The listing builds one solid part. Answer for the finished solid, in the listing's coordinates (mm). A direction names the side the tool comes from. Give positions to 0.01 mm unless a question says otherwise; leave off trailing zeros. Write each loop counter-clockwise with the first axis right and the second up, starting at its lowest first coordinate (ties: lowest second). Pieces come first, ordered by that corner, then holes. Notation, with made-up numbers: (43, 60) - (64, 60) arc R26 cw to (64, 99) - close; hole circle Ø4 at (14.25, 68.25). An arc over 180 degrees is marked (long way). Return JSON: item names as keys, results as strings.
from build123d import *

# Parameters (mm, degrees)
SKETCH1_W           = 340
SKETCH1_H           = 42.5
BOSS_EXTRUDE1_DEPTH = 41.5
SKETCH2_R           = 9.5
CUT_EXTRUDE1_DEPTH  = 10
SKETCH4_R           = 3.05
CUT_EXTRUDE3_DEPTH  = 301.787476707
CUT_EXTRUDE4_DEPTH  = 344.473796902


with BuildPart() as part:
    # Sketch1 → Boss-Extrude1 (new body)
    with BuildSketch(Plane(origin=(0, 0, 0), x_dir=(1, 0, 0), z_dir=(0, 1, 0))):
        with Locations((126.814516129, -4.284274194)):
            Rectangle(SKETCH1_W, SKETCH1_H)
    extrude(amount=BOSS_EXTRUDE1_DEPTH)

    # Sketch2 → Cut-Extrude1 (cut)
    with BuildSketch(Plane(origin=(0, 41.5, 0), x_dir=(1, 0, 0), z_dir=(0, 1, 0))):
        with Locations(Location((-5.685483871, -4.284274194, 0), (0, 0, 270))):
            Circle(SKETCH2_R)
        with Locations(Location((26.914516129, -4.284274194, 0), (0, 0, 270))):
            Circle(SKETCH2_R)
        with Locations(Location((59.514516129, -4.284274194, 0), (0, 0, 270))):
            Circle(SKETCH2_R)
        with Locations(Location((92.114516129, -4.284274194, 0), (0, 0, 270))):
            Circle(SKETCH2_R)
        with Locations(Location((124.714516129, -4.284274194, 0), (0, 0, 270))):
            Circle(SKETCH2_R)
        with Locations(Location((157.314516129, -4.284274194, 0), (0, 0, 270))):
            Circle(SKETCH2_R)
        with Locations(Location((189.914516129, -4.284274194, 0), (0, 0, 270))):
            Circle(SKETCH2_R)
        with Locations(Location((222.514516129, -4.284274194, 0), (0, 0, 270))):
            Circle(SKETCH2_R)
        with Locations(Location((255.114516129, -4.284274194, 0), (0, 0, 270))):
            Circle(SKETCH2_R)
    extrude(amount=-CUT_EXTRUDE1_DEPTH, mode=Mode.SUBTRACT)

    # Sketch4 → Cut-Extrude3 (cut, through all)
    with BuildSketch(Plane(origin=(0, 41.5, 0), x_dir=(1, 0, 0), z_dir=(0, 1, 0))):
        with Locations(Location((286.814516129, 8.965725806, 0), (0, 0, 90))):
            Circle(SKETCH4_R)
        with Locations(Location((-33.185483871, -17.534274194, 0), (0, 0, 90))):
            Circle(SKETCH4_R)
    extrude(amount=-CUT_EXTRUDE3_DEPTH, mode=Mode.SUBTRACT)

    # Sketch3 → Cut-Extrude4 (cut, through all)
    with BuildSketch(Plane.ZY.offset(43.185483871)):
        with BuildLine():
            Line((-6.965725806, 41.5), (-16.965725806, 41.5))
            Line((-16.965725806, 41.5), (-16.965725806, 31.5))
            ThreePointArc((-16.965725806, 31.5), (-14.036793618, 38.571067812), (-6.965725806, 41.5))
        make_face()
        with BuildLine():
            ThreePointArc((-6.965725806, 0), (-14.036793618, 2.928932188), (-16.965725806, 10))
            Line((-16.965725806, 10), (-16.965725806, 0))
            Line((-16.965725806, 0), (-6.965725806, 0))
        make_face()
        with BuildLine():
            Line((25.534274194, 0), (25.534274194, 10))
            ThreePointArc((25.534274194, 10), (22.605342005, 2.928932188), (15.534274194, 0))
            Line((15.534274194, 0), (25.534274194, 0))
        make_face()
        with BuildLine():
            Line((25.534274194, 41.5), (15.534274194, 41.5))
            ThreePointArc((15.534274194, 41.5), (22.605342005, 38.571067812), (25.534274194, 31.5))
            Line((25.534274194, 31.5), (25.534274194, 41.5))
        make_face()
    extrude(amount=-CUT_EXTRUDE4_DEPTH, mode=Mode.SUBTRACT)


solid = part.part
Item 1: A cutting plane is placed at C-C on y = 36. Give the number of separate pieces and of enclosed holes in the cut face, then the cut area to 3 significant figures.
Answer below:
{"separate pieces": "1", "enclosed holes": "11", "area": "11,100 mm²"}
Item 2: For faces 5 (the face through (50.24, 36.57, 2.22)), 6 (the face through (-30.48, 21.04, 16.13)), determine the directions among +Z, -Z, +X, -X, +Y, -Y from which every point of the face is accessible in a straight line to the end or side of a thin tool.
Answer below:
{"face 5": "+Y", "face 6": "+Y, -Y"}
Item 3: Flat-ended cylindrical pins translate along their axes: P1, Ø5.5, axis at x = 220.5, z = 6.5, coming from the +Y side; P2, Ø1, axis at x = 256.5, y = 7.5, coming from the +Z side. Find the tip coordinate at first contact, or state that the pin passes through.
Answer below:
{"P1": "stops at y = 31.5", "P2": "stops at z = 25.33"}
Item 4: The mould has two halves that part along X. Classify faces 1 (the face through (124, 21, -16.966)), 2 (the face through (100.125, 36.57, 9.391)), 3 (the face through (-43.185, 20, 5)), 4 (the face through (92, 31.5, 4)): +X half, -X half, draft (parallel to the pull), parting line (faces both ways), or undercut.
Answer below:
{"face 1": "draft", "face 2": "undercut", "face 3": "-X half", "face 4": "undercut"}
Item 5: A cutting plane is placed at D-D on x = 62.5. Determine the outline of the cut face in (y, z), then the cut area to 3 significant figures.
Answer below:
{"outline": "(0, -6.97) arc R10 ccw to (10, -16.97) - (31.5, -16.97) arc R10 ccw to (41.5, -6.97) - (41.5, -4.73) - (31.5, -4.73) - (31.5, 13.3) - (41.5, 13.3) - (41.5, 15.53) arc R10 ccw to (31.5, 25.53) - (10, 25.53) arc R10 ccw to (0, 15.53) - close", "area": "1,500 mm²"}
Item 6: Consider L1, parallel to Y at x = 257.5, z = 1.5; L2, parallel to Z at x = 253, y = 35; L3, parallel to X at y = 5.5, z = -11.5. Determine where each line is inside the solid, lowest interval first.
Answer below:
{"L1": "y = 0 to 31.5", "L2": "z = -16.33 to -4.98, 13.55 to 24.9", "L3": "x = -43.19 to 285.12, 288.51 to 296.81"}
Item 7: A cutting plane is placed at B-B on x = -12. Determine the outline of the cut face in (y, z), then the cut area to 3 significant figures.
Answer below:
{"outline": "(0, -6.97) arc R10 ccw to (10, -16.97) - (31.5, -16.97) arc R10 ccw to (41.5, -6.97) - (41.5, -2.81) - (31.5, -2.81) - (31.5, 11.38) - (41.5, 11.38) - (41.5, 15.53) arc R10 ccw to (31.5, 25.53) - (10, 25.53) arc R10 ccw to (0, 15.53) - close", "area": "1,540 mm²"}
Item 8: A cutting plane is placed at A-A on y = 4.5. Determine the outline of the cut face in (x, z).
Answer below:
{"outline": "(-43.19, -15.32) - (296.81, -15.32) - (296.81, 23.89) - (-43.19, 23.89) - close; hole circle Ø6.1 at (-33.19, 17.53); hole circle Ø6.1 at (286.81, -8.97)"}
